Geometry: final body of the model. Coordinates: model frame, mm. A direction names the side the tool comes from. Give positions to 0.01 mm unless a question says otherwise; leave off trailing zeros. Order: outer loops, then holes, each group sorted by start corner. A loop starts at its lowest first (then second) coordinate and runs counter-clockwise, first axis right, second up. Notation, with made-up numbers: (74.5, -6) -> (129.5, -6) arc R20 cw to (129.5, 16) -> close; hole circle Ø7 at (-22, 59.25). An arc over 180 degrees is marked (long way). Answer in a Markdown table with one row per item. Add a question column.
Q1. Pull-direction query (Y, two-part tool) for faces 3 (the face through (11.92, 0.62, -0.14)), 4 (the face through (0, 5, 0)), 5 (the face through (29.625, 2.319, -0.515)); classes: +Y half, -Y half, draft (parallel to the pull), parting line (faces both ways), or undercut.
Q2. Cut plane B-B on x = 17.25. Return the cut outline in (y, z), and give its area (3 significant figures).
Q3. Contact query for flat-ended pins moving along their axis: P1, Ø3, axis at x = 12, y = 4, coming from the -Z side; P2, Ø3, axis at x = 15, z = 6, coming from the +Y side; P3, Ø0.9, axis at y = 0, z = 4, coming from the -X side. Output: stop coordinate, or through.
Q4. Set-up query: faces 1 (the face through (10, 3.6, 2.1)), 2 (the face through (12.38, 7.81, -1.73)). Return all of +Z, -Z, +X, -X, +Y, -Y with unobstructed straight access to the full face (end or side cutting, diameter ignored); none if empty.
Q5. Line query: line 1 along Z through (x, y) = (2.25, 1.25); line 2 along Z through (x, y) = (4.25, -1); line 3 along Z through (x, y) = (18.75, 4). Output: solid intervals per line, ascending. Write a range as from..to.
Q6. Cut plane A-A on x = 26.75. Return the cut outline in (y, z), and give its area (3 significant figures).
from build123d import *

# Parameters (mm, degrees)
CUT_EXTRUDE_1_DEPTH = 10


with BuildPart() as part:
    # 草图1 → Revolve 543 (revolve)
    with BuildSketch(Plane.XY, mode=Mode.PRIVATE) as revolve_543_sk:
        Polygon((0, 0), (30, 0), (30, 2), (24, 8), (1.072, 8), (0, 6.928), align=None)
    revolve(revolve_543_sk.sketch.rotate(Axis((-1.4104518, 0, 0), (1, 0, 0)), 90), axis=Axis((-1.4104518, 0, 0), (1, 0, 0)))

    # 草图2 → 切除-拉伸1 (cut)
    with BuildSketch(Plane.ZY):
        Polygon((4.5745, 0), (2.28725, 3.96163321), (-2.28725, 3.96163321), (-4.5745, 0), (-2.28725, -3.96163321), (2.28725, -3.96163321), align=None)
    extrude(amount=-CUT_EXTRUDE_1_DEPTH, mode=Mode.SUBTRACT)

    # 草图3 → 切除-旋转1 (revolve, cut)
    with BuildSketch(Plane.XY, mode=Mode.PRIVATE) as cut_revolve_1_sk:
        Polygon((10, 3.96163321), (12.28725, 0), (10, 0), align=None)
    revolve(cut_revolve_1_sk.sketch.rotate(Axis((-0.121283255, 0, 0), (1, 0, 0)), 90), axis=Axis((-0.121283255, 0, 0), (1, 0, 0)), mode=Mode.SUBTRACT)


solid = part.part
Completed:
| question | item | result |
|---|---|---|
| 1 | face 3 | undercut |
| 1 | face 4 | draft |
| 1 | face 5 | parting line |
| 2 | outline | circle Ø16 at (0, 0) |
| 2 | area | 201 mm² |
| 3 | P1 | stops at z = -7.6 |
| 3 | P2 | stops at y = 6.61 |
| 3 | P3 | stops at x = 10 |
| 4 | face 1 | -X |
| 4 | face 2 | +X, -X |
| 5 | line 1 | z = -7.9..-3.85, 3.85..7.9 |
| 5 | line 2 | z = -7.94..-4, 4..7.94 |
| 5 | line 3 | z = -6.93..6.93 |
| 6 | outline | circle Ø10.5 at (0, 0) |
| 6 | area | 86.6 mm² |
